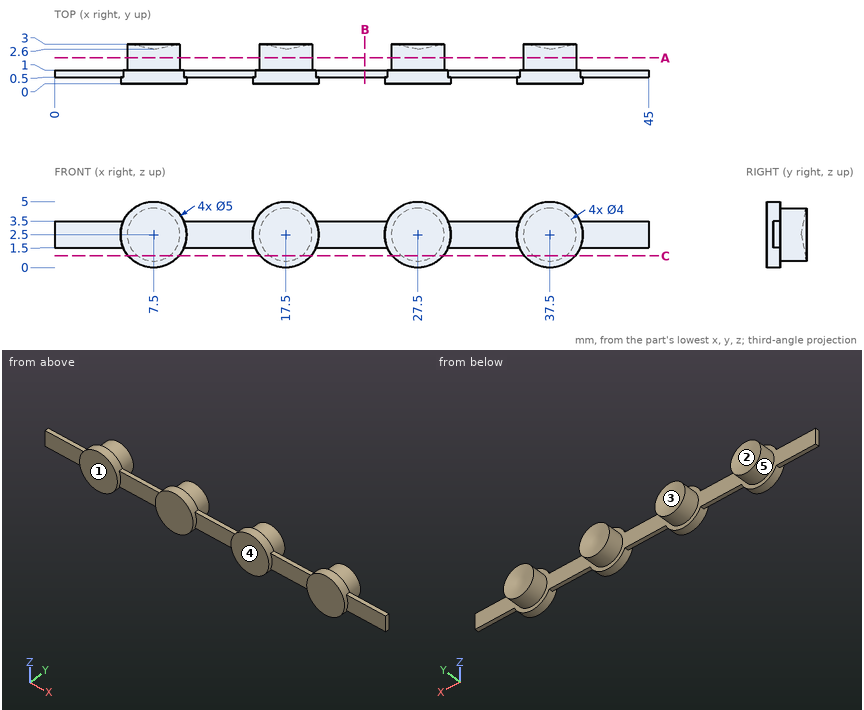
The figure shows three views and two pictorial views of one solid part (mm, origin at its lowest corner). Answer the questions. A direction names the side the tool comes from. Round coordinates to 2 decimals unless told otherwise and drop trailing zeros. Order: outer loops, then holes, each group sorted by start corner. A loop starts at its lowest first (then second) coordinate and runs counter-clockwise, first axis right, second up. Notation, with made-up numbers: (72.5, -26.75) -> (118.5, -26.75) arc R12 cw to (118.5, -10.75) -> close; hole circle Ø1 at (-37.5, 18.5). An arc over 180 degrees is marked (long way). Put each result on its own line as item: value.
Q1. Consider line 1 along X through (y, z) = (2.15, 1.4); line 2 along X through (y, z) = (2.8, 4); line 3 along Y through (x, z) = (22, 2). Determine where each line is inside the solid, lowest interval first.
Results list:
line 1: 5.83 to 9.17, 15.83 to 19.17, 25.83 to 29.17, 35.83 to 39.17
line 2: 6.18 to 8.82, 16.18 to 18.82, 26.18 to 28.82, 36.18 to 38.82
line 3: 0.5 to 1
Q2. Section A-A, the plane y = 1.95 is taken. Write down the section's boundary in (x, z), and give its area (3 significant figures).
Results list:
outline: circle Ø4 at (7.5, 2.5); circle Ø4 at (17.5, 2.5); circle Ø4 at (27.5, 2.5); circle Ø4 at (37.5, 2.5)
area: 50.3 mm^2
Q3. Determine the mould class of the marked faces 1, 2 and 3 for opening direction X: pulls with the +X half, pulls with the -X half, needs draft (parallel to the pull), parting line crosses it, or undercut.
Results list:
face 1: needs draft
face 2: undercut
face 3: undercut
Q4. Section B-B, the plane x = 23.5 is taken. Write down the section's boundary in (y, z).
Results list:
outline: (0.5, 1.5) -> (1, 1.5) -> (1, 3.5) -> (0.5, 3.5) -> close
Q5. Each of these flat-tipped pins is pushed along its axis until it touches: P1, Ø1, axis at x = 22.5, z = 2.5, coming from the -Y side; P2, Ø1, axis at x = 32.5, z = 0.5, coming from the +Y side; P3, Ø0.6, axis at x = 43, y = 1, coming from the +Z side; P4, Ø0.6, axis at x = 2, y = 1, coming from the -Z side. Where does it stop, or does it pass through?
Results list:
P1: y = 0.5
P2: through
P3: z = 3.5
P4: z = 1.5
Q6. Section C-C, the plane z = 0.9 is taken. Count the separate pieces of the cut face and the enclosed holes in it, and give its area (3 significant figures).
Results list:
separate pieces: 4
enclosed holes: 0
area: 34.1 mm^2
Q7. Which of the six approach directions +Z, -Z, +X, -X, +Y, -Y give full straight-line access (tool end or side, diameter ignored) to the marked faces 4 and 5?
Results list:
face 4: +Z, -Z, +X, -X, -Y
face 5: +Y
